```python
from build123d import *

# Parameters (mm, degrees)
SKETCH_1_R      = 30
EXTRUDE_1_DEPTH = 40
EXTRUDE_2_DEPTH = 15


with BuildPart() as part:
    # 草图1 → 凸台-拉伸1 (new body)
    with BuildSketch(Plane(origin=(0, 0, 0), x_dir=(1, 0, 0), z_dir=(0, 1, 0))):
        with Locations(Location((0, 0, 0), (0, 0, 270))):
            Circle(SKETCH_1_R)
    extrude(amount=EXTRUDE_1_DEPTH)

    # 草图2 → 凸台-拉伸2 (add, symmetric)
    with BuildSketch(Plane.XY):
        Polygon((-15, 40), (-15, 80), (-40, 40), align=None)
        Polygon((15, 40), (40, 40), (15, 80), align=None)
    extrude(amount=EXTRUDE_2_DEPTH, both=True)


solid = part.part
```
Check sheet for the modelled part. Datum: model origin and axes. Units: mm. A direction names the side the tool comes from. Give positions to 0.01 mm unless a question says otherwise; leave off trailing zeros. Order: outer loops, then holes, each group sorted by start corner. A loop starts at its lowest first (then second) coordinate and runs counter-clockwise, first axis right, second up. Notation, with made-up numbers: M -12,15.5 L 37,15.5 A25 ccw 37,36.5 Z; hole C -34,-22 d5. An arc over 180 degrees is marked long. Answer in a Markdown table with one row per item.
1) Gauge pin test, flat ends, axial feed: P1, Ø20, axis at x = -30, y = 64.5, coming from the +Z side; P2, Ø4, axis at x = -5.5, y = 17, coming from the -Z side; P3, Ø3, axis at y = 15, z = 12.5, coming from the +X side; P4, Ø8, axis at y = 71, z = -19.5, coming from the +X side. Record the tip position at first contact, or that the pin passes through.
Filled sheet:
| item | result |
|---|---|
| P1 | stops at z = 15 |
| P2 | stops at z = -29.8 |
| P3 | stops at x = 27.91 |
| P4 | passes through |
2) Thickness scan on L1, parallel to Y at x = -2, z = 17; L2, parallel to X at y = 32.5, z = -0.5; L3, parallel to Z at x = 15, y = 13. Record the ranges inside material, lowest first. Write a range as [from, to].
Filled sheet:
| item | result |
|---|---|
| L1 | y = [0, 40] |
| L2 | x = [-30, 30] |
| L3 | z = [-25.98, 25.98] |
3) Cross-section at A-A, the plane z = 0. Enter the section's corners in (x, y).
Filled sheet:
| item | result |
|---|---|
| outline | M -40,40 L -30,40 L -30,0 L 30,0 L 30,40 L 40,40 L 15,80 L 15,40 L -15,40 L -15,80 Z |
4) Cross-section at D-D, the plane z = 8.5. Enter the section's corners in (x, y), plus the area to 3 significant figures.
Filled sheet:
| item | result |
|---|---|
| outline | M -40,40 L -28.77,40 L -28.77,0 L 28.77,0 L 28.77,40 L 40,40 L 15,80 L 15,40 L -15,40 L -15,80 Z |
| area | 3,300 mm2 |
5) Release check for a two-part mould opening along X. For faces 1 (the flat face through (0, 0, 0)), 2 (the flat face through (-27.325, 60.28, -0.21)), 3 (the flat face through (-15, 60, 0)) record: +X half, -X half, draft (parallel to the pull), parting line (faces both ways), or undercut.
Filled sheet:
| item | result |
|---|---|
| face 1 | draft |
| face 2 | -X half |
| face 3 | undercut |
6) Cross-section at C-C, the plane x = 0. Enter the section's corners in (y, z).
Filled sheet:
| item | result |
|---|---|
| outline | M 0,-30 L 40,-30 L 40,30 L 0,30 Z |
7) Cross-section at B-B, the plane y = 61.5. Enter the section's corners in (x, z), plus the area to 3 significant figures.
Filled sheet:
| item | result |
|---|---|
| outline | M -26.56,-15 L -15,-15 L -15,15 L -26.56,15 Z; M 15,-15 L 26.56,-15 L 26.56,15 L 15,15 Z |
| area | 694 mm2 |
8) Access from +Z, -Z, +X, -X, +Y, -Y to the whole of each face (thin tool, end or side, straight path). Record for faces 4 (the flat face through (-22, 51, 15)), 5 (the flat face through (15, 60, 0)), 6 (the cylindrical face through (1.32, 19.72, -29.97)), 7 (the flat face through (22, 51, -15)).
Filled sheet:
| item | result |
|---|---|
| face 4 | +Z, +X, -X, +Y |
| face 5 | +Z, -Z, +Y |
| face 6 | -Y |
| face 7 | -Z, +X, -X, +Y |
